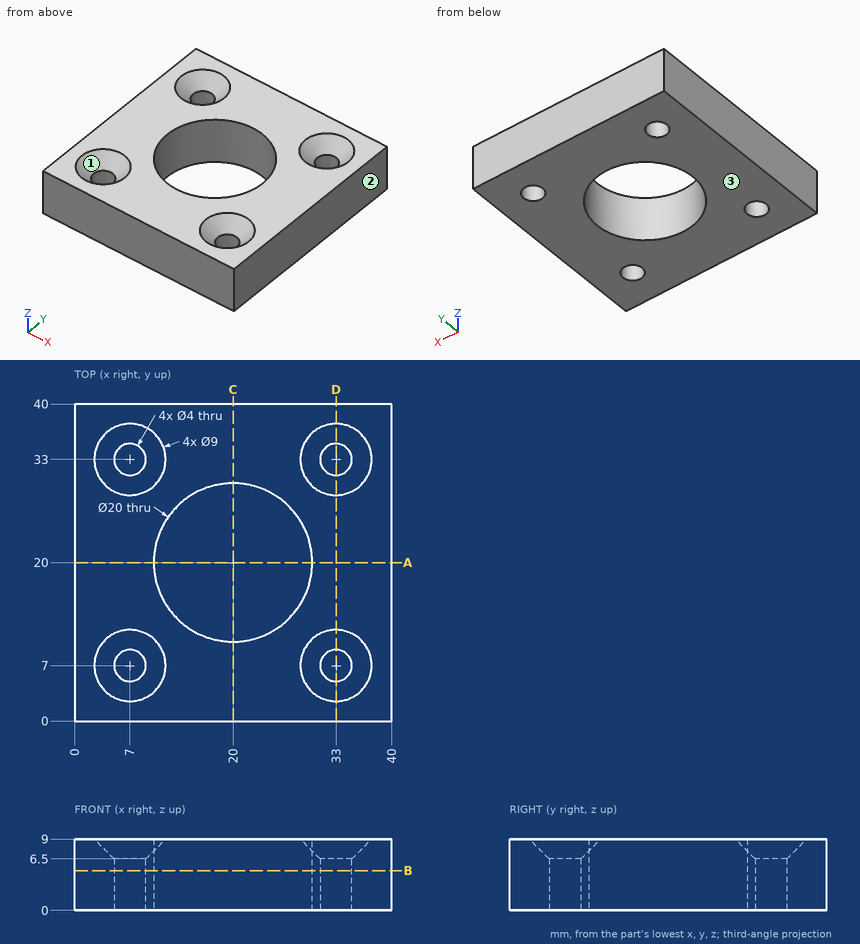
For this review, use the dimensioned drawing (mm, ordinates from the lowest corner) and the shaded views. Coordinates: 2 decimals unless noted, no trailing zeros. Order: outer loops, then holes, each group sorted by start corner. A loop starts at its lowest first (then second) coordinate and runs counter-clockwise, first axis right, second up. Notation, with made-up numbers: M 43.5,29 L 91.5,29 A31 cw 91.5,64 Z; hole C 1,33.25 d5. An arc over 180 degrees is marked long. Answer as a JSON object with one key per item and string values. Group by question number.
1) Mouldability with a two-part tool opening along X and no side actions: class the marked faces 1, 2 and 3 as pulls with the +X half, pulls with the -X half, needs draft (parallel to the pull), parting line crosses it, or undercut.
2) Add section A-A, the plane y = 20. Write out the cut boundary in (x, z).
3) Add section D-D, the plane x = 33. Write out the cut boundary in (y, z).
4) Wall thickness on L1, parallel to Y at x = 33, z = 1.75; L2, parallel to Y at x = 20, z = 6.5; L3, parallel to Y at x = 31.5, z = 8: over which ranges is each line inside the solid? List them lowest first.
5) Add section B-B, the plane z = 5. Write out the cut boundary in (x, y), then the cut area to 3 significant figures.
6) For pin 1 (5 mm diameter, centred on y = 29, z = 4.5, fed in from -X); pin 2 (5 mm diameter, centred on x = 33, y = 33, fed in from +Z); pin 3 (4.5 mm diameter, centred on x = 33, y = 7, fed in from +Z); pin 4 (1.5 mm diameter, centred on x = 6, y = 31, fed in from +Z), all flat-tipped, find the tip position at first contact; note any pin that passes through.
Computed values:
{
 "1": {"face 1": "undercut", "face 2": "pulls with the +X half", "face 3": "needs draft"},
 "2": {"outline": "M 0,0 L 10,0 L 10,9 L 0,9 Z; M 30,0 L 40,0 L 40,9 L 30,9 Z"},
 "3": {"outline": "M 0,0 L 5,0 L 5,6.5 L 2.5,9 L 0,9 Z; M 9,0 L 31,0 L 31,6.5 L 28.5,9 L 11.5,9 L 9,6.5 Z; M 35,0 L 40,0 L 40,9 L 37.5,9 L 35,6.5 Z"},
 "4": {"L1": "y = 0 to 5, 9 to 31, 35 to 40", "L2": "y = 0 to 10, 30 to 40", "L3": "y = 0 to 3.84, 10.16 to 29.84, 36.16 to 40"},
 "5": {"outline": "M 0,0 L 40,0 L 40,40 L 0,40 Z; hole C 7,7 d4; hole C 7,33 d4; hole C 20,20 d20; hole C 33,7 d4; hole C 33,33 d4", "area": "1,240 mm^2"},
 "6": {"pin 1": "stops at x = 0", "pin 2": "stops at z = 7", "pin 3": "stops at z = 6.75", "pin 4": "stops at z = 7.49"}
}
